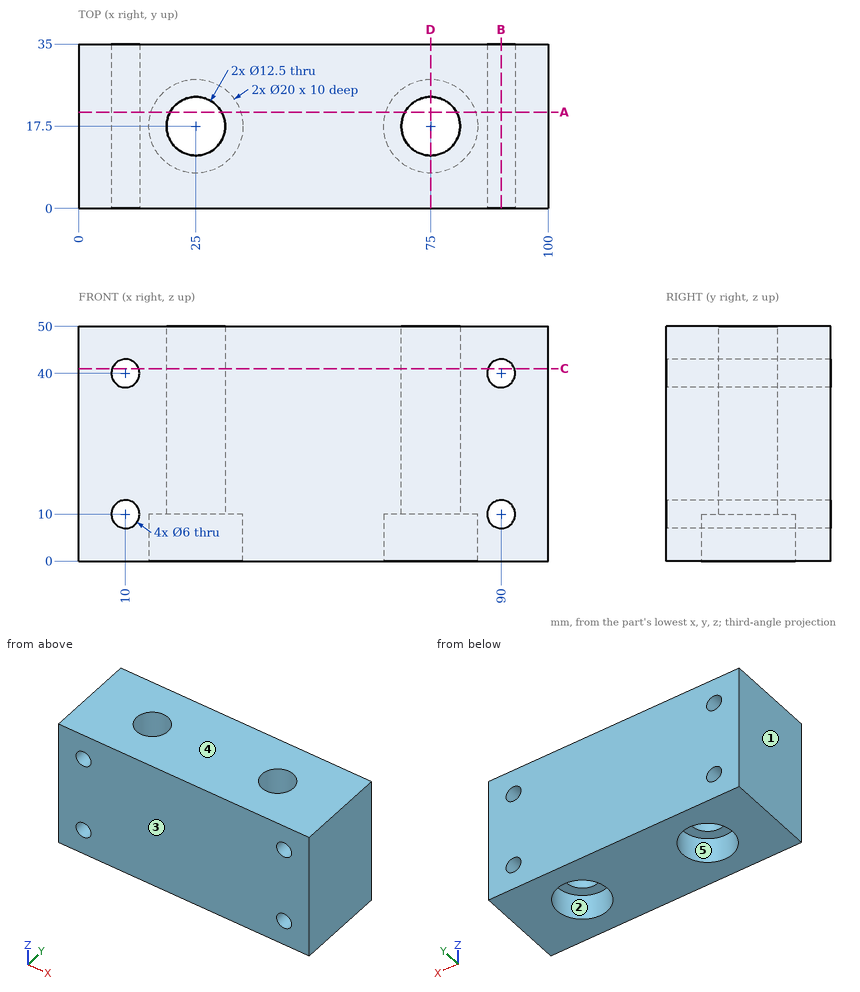
Design review of the part shown in the three views and the two pictorial views. Dimensions are in mm from the part's minimum x, y and z. A direction names the side the tool comes from. Coordinates: 2 decimals unless noted, no trailing zeros. Order: outer loops, then holes, each group sorted by start corner. A loop starts at its lowest first (then second) coordinate and runs counter-clockwise, first axis right, second up.
Item 1: Take a section at B-B, the plane x = 90. Write out the cut boundary in (y, z), then the cut area to 3 significant figures.
Item 2: For pin 1 Ø8 at (x, y) = (17.5, 8) entering from -Z; pin 2 Ø10 at (x, y) = (25, 17.5) entering from -Z; pin 3 Ø16 at (x, y) = (25, 17.5) entering from -Z, all flat-tipped, find the tip position at first contact; note any pin that passes through.
Item 3: Take a section at C-C, the plane z = 41. Write out the cut boundary in (x, y), then the cut area to 3 significant figures.
Item 4: For the marked faces 4 and 5, list the 3-axis set-ups (+Z, -Z, +X, -X, +Y, -Y) from which the entire face can be reached by the end or side of a thin tool; tool diameter is ignored.
Item 5: Take a section at A-A, the plane y = 20.5. Write out the cut boundary in (x, z), then the cut area to 3 significant figures.
Item 6: For line 1 (Z direction, x = 10, y = 31); line 2 (X direction, y = 17.5, z = 25.5); line 3 (Y direction, x = 75, z = 4), list the stretches that pass through material, from the lowest coordinate up.
Item 7: The part is to be moulded in two halves that separate along X. For the marked faces 1, 2 and 3, say which applies: pulls with the +X half, pulls with the -X half, needs draft (parallel to the pull), parting line crosses it, or undercut.
Item 8: Take a section at D-D, the plane x = 75. Write out the cut boundary in (y, z).
The answers:
1. outline: (0, 0) - (35, 0) - (35, 7) - (0, 7) - close; (0, 13) - (35, 13) - (35, 37) - (0, 37) - close; (0, 43) - (35, 43) - (35, 50) - (0, 50) - close
1. area: 1,330 mm2
2. pin 1: stops at z = 0
2. pin 2: passes through
2. pin 3: stops at z = 10
3. outline: (0, 0) - (7.17, 0) - (7.17, 35) - (0, 35) - close; (12.83, 0) - (87.17, 0) - (87.17, 35) - (12.83, 35) - close; (92.83, 0) - (100, 0) - (100, 35) - (92.83, 35) - close; hole circle Ø12.5 at (25, 17.5); hole circle Ø12.5 at (75, 17.5)
3. area: 2,860 mm2
4. face 4: +Z, +X, -X, +Y, -Y
4. face 5: -Z
5. outline: (0, 0) - (15.46, 0) - (15.46, 10) - (19.52, 10) - (19.52, 50) - (0, 50) - close; (30.48, 10) - (34.54, 10) - (34.54, 0) - (65.46, 0) - (65.46, 10) - (69.52, 10) - (69.52, 50) - (30.48, 50) - close; (80.48, 10) - (84.54, 10) - (84.54, 0) - (100, 0) - (100, 50) - (80.48, 50) - close; hole circle Ø6 at (10, 10); hole circle Ø6 at (10, 40); hole circle Ø6 at (90, 10); hole circle Ø6 at (90, 40)
5. area: 3,630 mm2
6. line 1: z = 0 to 7, 13 to 37, 43 to 50
6. line 2: x = 0 to 18.75, 31.25 to 68.75, 81.25 to 100
6. line 3: y = 0 to 7.5, 27.5 to 35
7. face 1: pulls with the -X half
7. face 2: undercut
7. face 3: needs draft
8. outline: (0, 0) - (7.5, 0) - (7.5, 10) - (11.25, 10) - (11.25, 50) - (0, 50) - close; (23.75, 10) - (27.5, 10) - (27.5, 0) - (35, 0) - (35, 50) - (23.75, 50) - close
